Work out the finished part from the listing and answer in its coordinate system (mm). Face numbers are marked on the shaded views. A direction names the side the tool comes from. Coordinates: 2 decimals unless noted, no trailing zeros. Write each loop counter-clockwise with the first axis right and the second up, starting at its lowest first coordinate (ties: lowest second). Pieces come first, ordered by that corner, then holes. Notation, with made-up numbers: (17, -36.5) - (27, -36.5) arc R11 cw to (27, -24.5) - close; hole circle Ø7 at (-39.75, -31.5). An arc over 180 degrees is marked (long way). One line per item, written item: value.
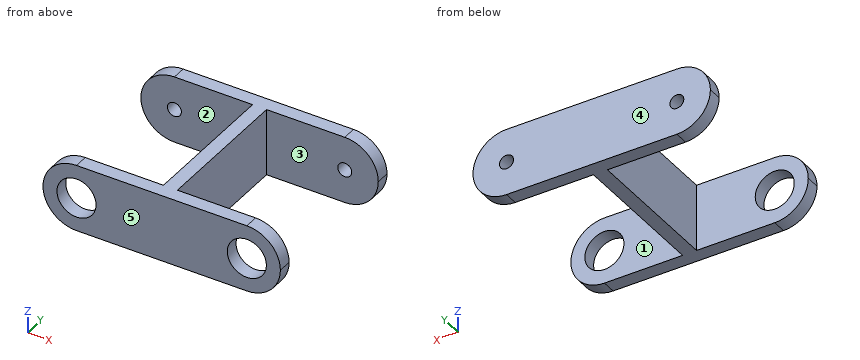
Autodesk Inventor part; units mm, degrees
ref_plane "YZ Plane" through (0, 0, 0) normal (1, 0, 0) x (0, 1, 0)
ref_plane "XZ Plane" through (0, 0, 0) normal (0, 1, 0) x (-1, 0, 0)
ref_plane "XY Plane" through (0, 0, 0) normal (0, 0, 1) x (1, 0, 0)
sketch "Sketch3" plane through (0, 0, 0) normal (0, 1, 0) x (-1, 0, 0)
  line L0 (2.5, 12) -> (-2.5, 12)
  line L1 (-2.5, 12) -> (-2.5, -12)
  line L2 (-2.5, -12) -> (2.5, -12)
  line L3 (2.5, -12) -> (2.5, 12)
  point P0 (0, 0)
  point P1 (0, 12)
  point P2 (2.5, 0)
  dimension "d6" = 5
  dimension "d7" = 24
extrude "Extrusion3" add sketch "Sketch3" along normal blind 61
sketch "Sketch4" plane through (2.5, 0, 12) normal (1, 0, 0) x (0, 0, -1)
  line L0 (0, 61) -> (24, 61)
  line L1 (24, 61) -> (24, 56)
  line L2 (24, 56) -> (0, 56)
  line L3 (0, 56) -> (0, 61)
  line L4 (0, 5) -> (24, 5)
  line L5 (24, 5) -> (24, 0)
  line L6 (24, 0) -> (0, 0)
  line L7 (0, 0) -> (0, 5)
  line L8 (0, 61) -> (24, 61)
  line L9 (0, 0) -> (24, 0)
  line L10 (0, 0) -> (0, 61)
  point P0 (12, 0)
  point P1 (12, 61)
  point P2 (12, 0)
  point P3 (12, 56)
  point P4 (12, 61)
  point P5 (12, 5)
  point P6 (12, 0)
  point P7 (0, 58.5)
  dimension "d10" = 5
extrude "Extrusion4" add sketch "Sketch4" along normal blind 40 and the other way blind 45
fillet "Fillet4" radius 12 8 edges at (42.5, 2.5, -12) (42.5, 2.5, 12) (42.5, 58.5, 12) (42.5, 58.5, -12) (-42.5, 58.5, 12) (-42.5, 2.5, 12) (-42.5, 58.5, -12) (-42.5, 2.5, -12)
sketch "Sketch8" plane through (0, 61, 0) normal (0, 1, 0) x (1, 0, 0)
  circle A0 centre (-30.5, 0) radius 2.5
  circle A1 centre (30.5, 0) radius 2.5
  arc A2 (-30.5, 12) -> (-30.5, -12) centre (-30.5, 0) ccw
  arc A3 (30.5, -12) -> (30.5, 12) centre (30.5, 0) ccw
  point P0 (0, 0)
  dimension "d27" = 5
extrude "Extrusion7" cut sketch "Sketch8" against normal up to surface (5 mm away)
sketch "Sketch9" plane through (0, 0, 0) normal (0, -1, 0) x (1, 0, 0)
  circle A0 centre (-30.5, 0) radius 7
  circle A1 centre (30.5, 0) radius 7
  arc A2 (-30.5, 12) -> (-30.5, -12) centre (-30.5, 0) ccw
  arc A3 (30.5, -12) -> (30.5, 12) centre (30.5, 0) ccw
  point P0 (0, 0)
  dimension "d30" = 14
extrude "Extrusion8" cut sketch "Sketch9" against normal up to next
equation "\"d6\" = b_mat_thickness"
equation "\"d7\" = sa_diameter"
equation "\"d8\" = sa_thickness + s_height + s_shaft_height + 3 * b_mat_thickness"
equation "\"d10\" = b_mat_thickness"
equation "\"d24\" = d11 + b_mat_thickness"
equation "\"d26\" = 0.5 * sa_diameter"
equation "\"d30\" = bb_outer_diameter"
properties part number "Middle_leg"
Item 1: Determine the mould class of the marked faces 3, 4 and 5 for opening direction Y: +Y half, -Y half, draft (parallel to the pull), parting line (faces both ways), or undercut.
Evaluation:
face 3: undercut
face 4: +Y half
face 5: -Y half
Item 2: Section C-C, the plane x = -36.5 is taken. Determine the outline of the cut face in (y, z).
Evaluation:
outline: (0, -10.39) - (5, -10.39) - (5, -3.61) - (0, -3.61) - close; (0, 3.61) - (5, 3.61) - (5, 10.39) - (0, 10.39) - close; (56, -10.39) - (61, -10.39) - (61, 10.39) - (56, 10.39) - close
Item 3: Section A-A, the plane x = 20 is taken. Determine the outline of the cut face in (y, z), then the cut area to 3 significant figures.
Evaluation:
outline: (0, -12) - (5, -12) - (5, 12) - (0, 12) - close; (56, -12) - (61, -12) - (61, 12) - (56, 12) - close
area: 240 mm2
Item 4: Which of the six approach directions +Z, -Z, +X, -X, +Y, -Y give full straight-line access (tool end or side, diameter ignored) to the marked faces 1 and 2?
Evaluation:
face 1: +Z, -Z, +X
face 2: +Z, -Z, -X
Item 5: Section D-D, the plane z = 4.5 is taken. Determine the outline of the cut face in (x, y).
Evaluation:
outline: (-41.62, 0) - (-35.86, 0) - (-35.86, 5) - (-41.62, 5) - close; (-41.62, 56) - (-2.5, 56) - (-2.5, 5) - (-25.14, 5) - (-25.14, 0) - (25.14, 0) - (25.14, 5) - (2.5, 5) - (2.5, 56) - (41.62, 56) - (41.62, 61) - (-41.62, 61) - close; (35.86, 0) - (41.62, 0) - (41.62, 5) - (35.86, 5) - close
Item 6: Given pin 1 (8 mm diameter, centred on y = 16, z = 7, fed in from -X), flat-ended and moving along its own axis, determine where the tip first touches the part or whether it passes through.
Evaluation:
pin 1: stops at x = -2.5
Item 7: Consider probe 1 along X at (y, z) = (57.95, 0); probe 2 along Y at (x, z) = (27, -6.25); probe 3 along Z at (x, y) = (-30.5, 58.3). Determine where each line is inside the solid, lowest interval first.
Evaluation:
probe 1: x = -42.5 to -33, -28 to 28, 33 to 42.5
probe 2: y = 0 to 5, 56 to 61
probe 3: z = -12 to -2.5, 2.5 to 12
Item 8: Section B-B, the plane z = -5 is taken. Determine the outline of the cut face in (x, y), then the cut area to 3 significant figures.
Evaluation:
outline: (-41.41, 0) - (-35.4, 0) - (-35.4, 5) - (-41.41, 5) - close; (-41.41, 56) - (-2.5, 56) - (-2.5, 5) - (-25.6, 5) - (-25.6, 0) - (25.6, 0) - (25.6, 5) - (2.5, 5) - (2.5, 56) - (41.41, 56) - (41.41, 61) - (-41.41, 61) - close; (35.4, 0) - (41.41, 0) - (41.41, 5) - (35.4, 5) - close
area: 985 mm2
